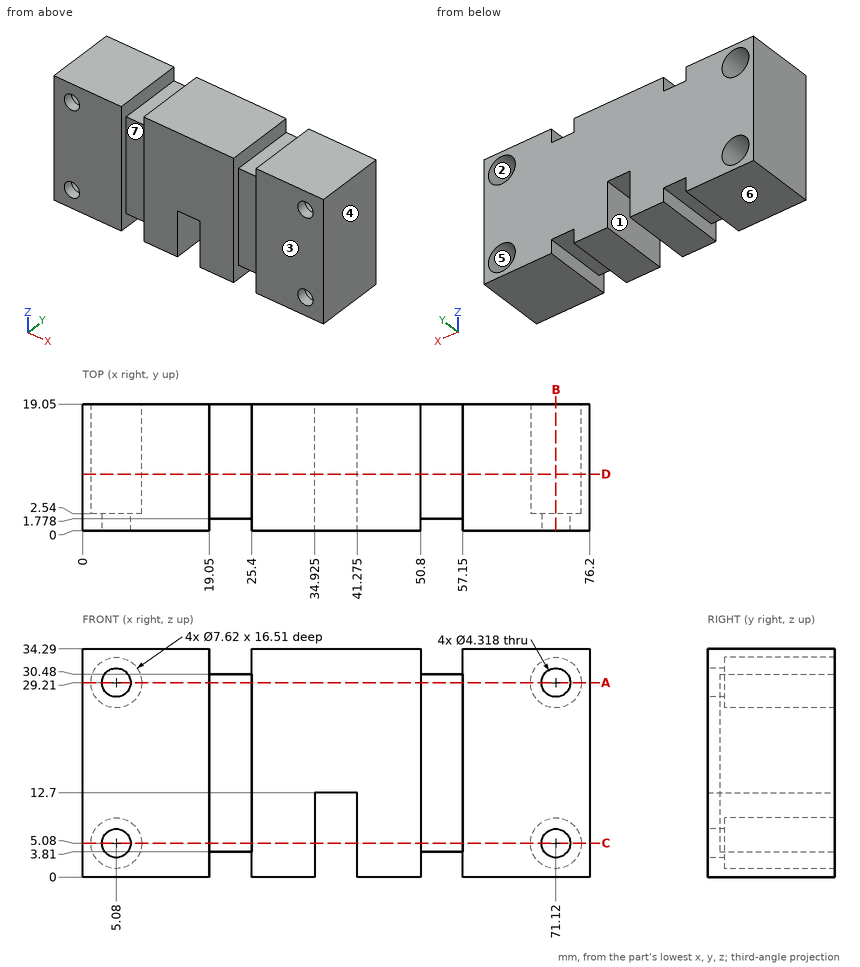
Here's the drawing with two shaded views (mm, measured from the low corner). I have some questions. A direction names the side the tool comes from. Coordinates: 2 decimals unless noted, no trailing zeros. Loops run counter-clockwise (first coordinate to the right, second up) from the corner with the lowest first, then second, coordinate; pieces in that order, holes last. Notation, with made-up numbers: (-24, 79.5) -> (-20, 79.5) arc R26 ccw to (-20, 115.5) -> close; hole circle Ø3 at (-23, -33.75). An arc over 180 degrees is marked (long way). Use one line per item in the form item = value. Start each with the question number.
(1) If we section it at C-C (z = 5.08): Give the number of separate pieces and of enclosed holes in the cut face, then the cut area to 3 significant figures.
(2) We'd pull the mould along X, two halves only. Please class the marked faces 1, 2, 3 and 4: pulls with the +X half, pulls with the -X half, needs draft (parallel to the pull), parting line crosses it, or undercut.
(3) On a 3-axis mill with a long thin cutter (end or side, diameter ignored), from which of +Z, -Z, +X, -X, +Y, -Y can I reach the whole of each face in a straight line? I mean the marked faces 5, 6 and 7. Say none if no direction works.
(4) If we section it at A-A (z = 29.21): Please give me the cut outline in (x, y), then the cut area to 3 significant figures.
(5) Please list where these lines run through material, in increasing order: line 1 along Z through (x, y) = (71.12, 1.9); line 2 along X through (y, z) = (1.5, 12.5) (3 decimals); line 3 along Z through (x, y) = (71.12, 13).
(6) Will these pins go through, and if not, where does the flat tip stop? pin 1 (1.9 mm diameter, centred on x = 54.5, z = 15.5, fed in from -Y); pin 2 (7 mm diameter, centred on x = 71.12, z = 5.08, fed in from +Y); pin 3 (3.5 mm diameter, centred on x = 71.12, z = 29.21, fed in from +Y); pin 4 (1.9 mm diameter, centred on x = 55.5, y = 10.5, fed in from -Z).
(7) If we section it at D-D (y = 8.5): Please give me the cut outline in (x, z) (3 decimals).
(8) If we section it at B-B (x = 71.12): Please give me the cut outline in (y, z), then the cut area to 3 significant figures.
Verdict:
q1.separate_pieces = 4
q1.enclosed_holes = 0
q1.area = 1,030 mm²
q2.face_1 = undercut
q2.face_2 = undercut
q2.face_3 = needs draft
q2.face_4 = pulls with the +X half
q3.face_5 = +Y
q3.face_6 = -Z, +X, -X, +Y, -Y
q3.face_7 = +Z, -Z, -Y
q4.outline = (0, 0) -> (2.92, 0) -> (2.92, 2.54) -> (1.27, 2.54) -> (1.27, 19.05) -> (0, 19.05) -> close; (7.24, 0) -> (19.05, 0) -> (19.05, 1.78) -> (25.4, 1.78) -> (25.4, 0) -> (50.8, 0) -> (50.8, 1.78) -> (57.15, 1.78) -> (57.15, 0) -> (68.96, 0) -> (68.96, 2.54) -> (67.31, 2.54) -> (67.31, 19.05) -> (8.89, 19.05) -> (8.89, 2.54) -> (7.24, 2.54) -> close; (73.28, 0) -> (76.2, 0) -> (76.2, 19.05) -> (74.93, 19.05) -> (74.93, 2.54) -> (73.28, 2.54) -> close
q4.area = 1,160 mm²
q5.line_1 = 0 to 2.92, 7.24 to 27.05, 31.37 to 34.29
q5.line_2 = 0 to 19.05, 25.4 to 34.925, 41.275 to 50.8, 57.15 to 76.2
q5.line_3 = 0 to 1.27, 8.89 to 25.4, 33.02 to 34.29
q6.pin_1 = 1.78
q6.pin_2 = 2.54
q6.pin_3 = through
q6.pin_4 = 3.81
q7.outline = (0, 0) -> (19.05, 0) -> (19.05, 3.81) -> (25.4, 3.81) -> (25.4, 0) -> (34.925, 0) -> (34.925, 12.7) -> (41.275, 12.7) -> (41.275, 0) -> (50.8, 0) -> (50.8, 3.81) -> (57.15, 3.81) -> (57.15, 0) -> (76.2, 0) -> (76.2, 34.29) -> (57.15, 34.29) -> (57.15, 30.48) -> (50.8, 30.48) -> (50.8, 34.29) -> (25.4, 34.29) -> (25.4, 30.48) -> (19.05, 30.48) -> (19.05, 34.29) -> (0, 34.29) -> close; hole circle Ø7.62 at (5.08, 5.08); hole circle Ø7.62 at (5.08, 29.21); hole circle Ø7.62 at (71.12, 5.08); hole circle Ø7.62 at (71.12, 29.21)
q8.outline = (0, 0) -> (19.05, 0) -> (19.05, 1.27) -> (2.54, 1.27) -> (2.54, 2.92) -> (0, 2.92) -> close; (0, 7.24) -> (2.54, 7.24) -> (2.54, 8.89) -> (19.05, 8.89) -> (19.05, 25.4) -> (2.54, 25.4) -> (2.54, 27.05) -> (0, 27.05) -> close; (0, 31.37) -> (2.54, 31.37) -> (2.54, 33.02) -> (19.05, 33.02) -> (19.05, 34.29) -> (0, 34.29) -> close
q8.area = 380 mm²
